CAD build for the part. Positions are in the model's coordinates, mm. A direction names the side the tool comes from. Give positions to 0.01 mm unless a question says otherwise; leave off trailing zeros. Order: outer loops, then holes, each group sorted by start corner. A loop starts at its lowest first (then second) coordinate and runs counter-clockwise, first axis right, second up. Notation, with made-up numbers: (-7, -34.75) -> (50, -34.75) arc R20 cw to (50, 4.25) -> close; hole circle Ø1 at (18.5, 30.25). An arc over 180 degrees is marked (long way). Use one line per item in the form item = value. Start each with the question number.
1) Drop flat-ended pins along their axis: P1, Ø5, axis at y = -14, z = 214.5, coming from the +X side; P2, Ø5, axis at x = 205, y = -11.5, coming from the -Z side; P3, Ø6, axis at x = -169.5, y = -22, coming from the -Z side; P4, Ø6, axis at x = -103, y = -131, coming from the +Z side. Give the stop position or say it passes through.
2) Cut at B-B, the plane z = 0. Give the cut face in (x, y).
3) Cut at A-A, the plane y = -9.5. Give the cut face in (x, z).
4) Probe line 1 (Z direction, x = -185.5, y = -112); line 2 (X direction, y = -36, z = 213); line 3 (Y direction, x = -69.5, z = -164.5). List the from-to ranges inside material, lowest first.
5) Tool access for faces 5 (the face through (94.5, -10, 161)), 6 (the face through (-172, -81, 67.31)), 7 (the face through (250.4, -20, 18)), 8 (the face through (212, -19, 216)), 9 (the face through (127, -10, 138.4)): list every direction of +Z, -Z, +X, -X, +Y, -Y with a clear straight run to the whole face (end or side of a thin tool).
6) Cut at C-C, the plane x = 80.5. Give the cut face in (y, z).
7) Cut at D-D, the plane z = 101. Give the cut face in (x, y), and give its area (3 significant figures).
8) Mould opens along Z. For faces 1 (the face through (127, -10, 238.4)), 2 (the face through (212, -10, 183.4)), 3 (the face through (179.5, -10, 161)), 4 (the face through (212, -10, 193.4)) say: pulls with the +Z half, pulls with the -Z half, needs draft (parallel to the pull), parting line crosses it, or undercut.
from build123d import *

# Parameters (mm, degrees)
F0_W     = 533.4
F0_H     = 533.4
F1_DEPTH = 2
F2_W     = 292.1
F2_H     = 184.15
F3_DEPTH = 35.814
F4_W     = 65
F4_H     = 45
F5_DEPTH = 17
F6_W     = 129.54
F6_H     = 170.18
F7_DEPTH = 160.02


with BuildPart() as f1:
    # F0 (on Front) → F1 (new body)
    with BuildSketch(Plane.XZ):
        Rectangle(F0_W, F0_H)
    extrude(amount=F1_DEPTH)

    # F2 (on face) → F3 (join)
    with BuildSketch(Plane.XZ.offset(2)):
        with Locations((104.35, 19.375)):
            Rectangle(F2_W, F2_H)
    extrude(amount=F3_DEPTH)

    # F4 (on face) → F5 (join)
    with BuildSketch(Plane.XZ.offset(2)):
        with Locations((127, 215.9)):
            Rectangle(F4_W, F4_H)
        with Locations((127, 160.9)):
            Rectangle(F4_W, F4_H)
        with Locations((212, 160.9)):
            Rectangle(F4_W, F4_H)
        with Locations((212, 215.9)):
            Rectangle(F4_W, F4_H)
    extrude(amount=F5_DEPTH)

    # F6 (on face) → F7 (join)
    with BuildSketch(Plane.XZ.offset(2)):
        with Locations((-171.45, 152.4)):
            Rectangle(F6_W, F6_H)
    extrude(amount=F7_DEPTH)


solid = f1.part
Result:
q1.P1 = 244.5
q1.P2 = -72.7
q1.P3 = 67.31
q1.P4 = through
q2.outline = (-266.7, -2) -> (-41.7, -2) -> (-41.7, -37.81) -> (250.4, -37.81) -> (250.4, -2) -> (266.7, -2) -> (266.7, 0) -> (-266.7, 0) -> close
q3.outline = (-236.22, 67.31) -> (-106.68, 67.31) -> (-106.68, 237.49) -> (-236.22, 237.49) -> close; (-41.7, -72.7) -> (250.4, -72.7) -> (250.4, 111.45) -> (-41.7, 111.45) -> close; (94.5, 138.4) -> (159.5, 138.4) -> (159.5, 183.4) -> (94.5, 183.4) -> close; (94.5, 193.4) -> (159.5, 193.4) -> (159.5, 238.4) -> (94.5, 238.4) -> close; (179.5, 138.4) -> (244.5, 138.4) -> (244.5, 183.4) -> (179.5, 183.4) -> close; (179.5, 193.4) -> (244.5, 193.4) -> (244.5, 238.4) -> (179.5, 238.4) -> close
q4.line_1 = 67.31 to 237.49
q4.line_2 = -236.22 to -106.68
q4.line_3 = -2 to 0
q5.face_5 = +Z, -Y
q5.face_6 = -Z, -X, -Y
q5.face_7 = +Z, -Z, +X, -Y
q5.face_8 = +Z, +X, -Y
q5.face_9 = +X, -Y
q6.outline = (-37.81, -72.7) -> (-2, -72.7) -> (-2, -266.7) -> (0, -266.7) -> (0, 266.7) -> (-2, 266.7) -> (-2, 111.45) -> (-37.81, 111.45) -> close
q7.outline = (-266.7, -2) -> (-236.22, -2) -> (-236.22, -162.02) -> (-106.68, -162.02) -> (-106.68, -2) -> (-41.7, -2) -> (-41.7, -37.81) -> (250.4, -37.81) -> (250.4, -2) -> (266.7, -2) -> (266.7, 0) -> (-266.7, 0) -> close
q7.area = 32,300 mm²
q8.face_1 = pulls with the +Z half
q8.face_2 = undercut
q8.face_3 = needs draft
q8.face_4 = undercut
